```python
from build123d import *

# Parameters (mm, degrees)
CROQUIS1_R                       = 4
SALIENTE_EXTRUIR1_DEPTH          = 35
CROQUIS2_R                       = 2
CORTAR_EXTRUIR1_DEPTH            = 10
TALADRO_DE_MARGEN_PARA_M31_D     = 3.4
TALADRO_DE_MARGEN_PARA_M31_DEPTH = 3
TALADRO_DE_MARGEN_PARA_M31_TIP   = 1.021463052


with BuildPart() as part:
    # Croquis1 → Saliente-Extruir1 (new body)
    with BuildSketch(Plane(origin=(0, 0, 0), x_dir=(1, 0, 0), z_dir=(0, 1, 0))):
        Circle(CROQUIS1_R)
    extrude(amount=SALIENTE_EXTRUIR1_DEPTH)

    # Croquis2 → Cortar-Extruir1 (cut)
    with BuildSketch(Plane(origin=(0, 35, 0), x_dir=(1, 0, 0), z_dir=(0, 1, 0))):
        Circle(CROQUIS2_R)
    extrude(amount=-CORTAR_EXTRUIR1_DEPTH, mode=Mode.SUBTRACT)

    # Taladro de margen para M31
    with Locations(Plane(origin=(-4, 32, 0), x_dir=(0, 0, -1), z_dir=(-1, 0, 0))):
        with Locations((0, 0)):
            Hole(TALADRO_DE_MARGEN_PARA_M31_D / 2, depth=TALADRO_DE_MARGEN_PARA_M31_DEPTH)
            with Locations((0, 0, -(TALADRO_DE_MARGEN_PARA_M31_DEPTH + TALADRO_DE_MARGEN_PARA_M31_TIP / 2))):  # 118° drill point
                Cone(0, TALADRO_DE_MARGEN_PARA_M31_D / 2, TALADRO_DE_MARGEN_PARA_M31_TIP, mode=Mode.SUBTRACT)


solid = part.part
```
The model under review builds one solid part; all positions refer to its coordinate system, in mm. A direction names the side the tool comes from. Round coordinates to 2 decimals unless told otherwise and drop trailing zeros. Loops run counter-clockwise (first coordinate to the right, second up) from the corner with the lowest first, then second, coordinate; pieces in that order, holes last. Notation, with made-up numbers: (24, 4.25) - (45, 4.25) arc R32 cw to (45, 34.25) - close; hole circle Ø6 at (-17.5, -40). An arc over 180 degrees is marked (long way). Use a Markdown table: item, result. Add a question column.
Q1. Add section A-A (z = 0). State the section outline as (x, y) points.
Q2. Add section B-B (y = 27.5). State the section outline as (x, z) points, plus the area to 3 significant figures.
Q3. For probe 1 along Z at (x, y) = (0, 29.5); probe 2 along Y at (x, z) = (-0.75, 0.5); probe 3 along Z at (x, y) = (-0.25, 15), list the stretches that pass through material, from the lowest coordinate up.
Q4. The part is to be moulded in two halves that separate along Z. For faces 3 (the face through (3.695, 17.255, 1.532)), 4 (the face through (-2.51, 32.65, 1.57)), 5 (the face through (0, 0, 0)), say which applies: pulls with the +Z half, pulls with the -Z half, needs draft (parallel to the pull), parting line crosses it, or undercut.
Q5. Add section C-C (x = 0). State the section outline as (y, z) points, plus the area to 3 significant figures.
Q6. Machinability: for faces 1 (the face through (-2, 35, 1)), 2 (the face through (0, 25, 0)), which of the approach directions +Z, -Z, +X, -X, +Y, -Y give a long, thin tool a straight path to every point of the face, cutting with its end or side? Answer none if there is none.
Q7. Add section D-D (x = -2.5). State the section outline as (y, z) points.
Q8. Insertion check: pin 1 Ø1.5 at (y, z) = (25, -1) entering from -X; pin 2 Ø1.5 at (y, z) = (13, -2.5) entering from -X; pin 3 Ø1.5 at (y, z) = (25.5, 3) entering from +X. Each pin has a flat end and moves straight along its axis. Give the tip position at first contact, or say it passes through.
Worked answers:
| question | item | result |
|---|---|---|
| 1 | outline | (-4, 0) - (4, 0) - (4, 35) - (2, 35) - (2, 25) - (-2, 25) - (-2, 30.3) - (-4, 30.3) - close; (-4, 33.7) - (-2, 33.7) - (-2, 35) - (-4, 35) - close |
| 2 | outline | circle Ø8 at (0, 0); hole circle Ø4 at (0, 0) |
| 2 | area | 37.7 mm² |
| 3 | probe 1 | -4 to -2, 2 to 4 |
| 3 | probe 2 | 0 to 25 |
| 3 | probe 3 | -3.99 to 3.99 |
| 4 | face 3 | parting line crosses it |
| 4 | face 4 | undercut |
| 4 | face 5 | needs draft |
| 5 | outline | (0, -4) - (35, -4) - (35, -2) - (25, -2) - (25, 2) - (35, 2) - (35, 4) - (0, 4) - close |
| 5 | area | 240 mm² |
| 6 | face 1 | +Z, -Z, +X, -X, +Y |
| 6 | face 2 | +Y |
| 7 | outline | (0, -3.12) - (35, -3.12) - (35, 3.12) - (0, 3.12) - close; hole circle Ø3.4 at (32, 0) |
| 8 | pin 1 | x = -3.99 |
| 8 | pin 2 | x = -3.6 |
| 8 | pin 3 | x = 3.31 |
